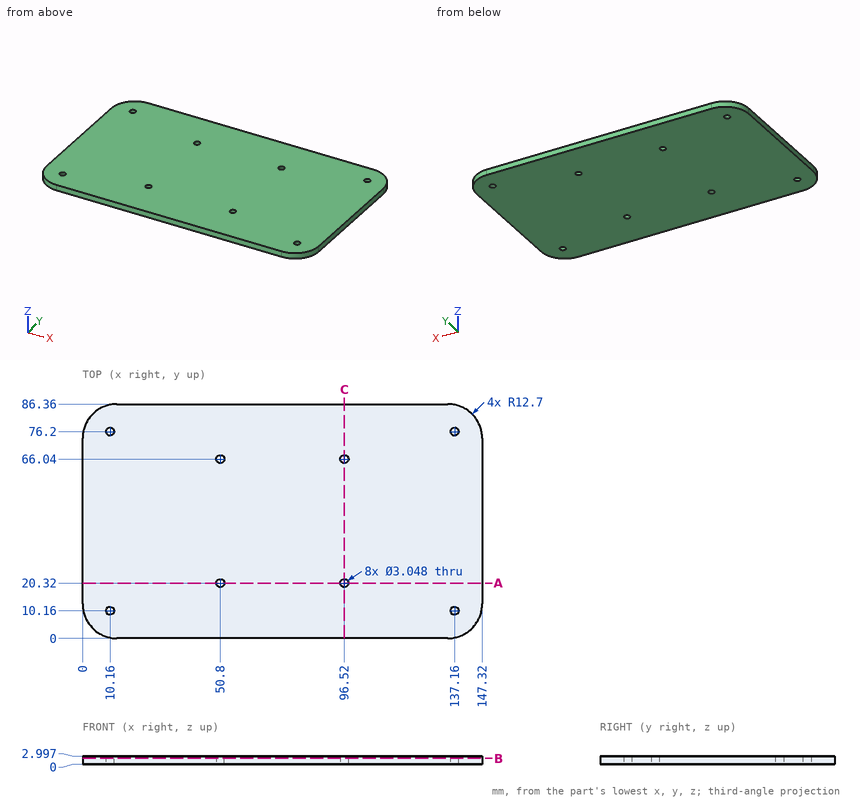
Answer from the drawing. Dimensions are ordinates in mm from the lowest x, y and z of the part. Round coordinates to 2 decimals unless told otherwise and drop trailing zeros. Loops run counter-clockwise (first coordinate to the right, second up) from the corner with the lowest first, then second, coordinate; pieces in that order, holes last.
1) A cutting plane is placed at B-B on z = 2.2. Give the number of separate pieces and of enclosed holes in the cut face, plus the area to 3 significant figures.
Outcome:
separate pieces: 1
enclosed holes: 8
area: 12,500 mm2
2) Given P1, Ø2.5, axis at x = 10.16, y = 76.2, coming from the +Z side; P2, Ø4, axis at x = 50.8, y = 66.04, coming from the -Z side, each flat-ended and moving along its own axis, determine where each tip first touches the part or whether it passes through.
Outcome:
P1: passes through
P2: stops at z = 0
3) Consider line 1 (Y direction, x = 50.8, z = 0.8); line 2 (X direction, y = 66.04, z = 1.5); line 3 (Y direction, x = 137, z = 1.85) (1 decimal). Determine where each line is inside the solid, lowest interval first.
Outcome:
line 1: y = 0 to 18.8, 21.84 to 64.52, 67.56 to 86.36
line 2: x = 0 to 49.28, 52.32 to 95, 98.04 to 147.32
line 3: y = 0.2 to 8.6, 11.7 to 74.7, 77.7 to 86.1
4) A cutting plane is placed at A-A on y = 20.32. Determine the outline of the cut face in (x, z), plus the area to 3 significant figures.
Outcome:
outline: (0, 0) - (49.28, 0) - (49.28, 3) - (0, 3) - close; (52.32, 0) - (95, 0) - (95, 3) - (52.32, 3) - close; (98.04, 0) - (147.32, 0) - (147.32, 3) - (98.04, 3) - close
area: 423 mm2
5) A cutting plane is placed at C-C on x = 96.52. Determine the outline of the cut face in (y, z).
Outcome:
outline: (0, 0) - (18.8, 0) - (18.8, 3) - (0, 3) - close; (21.84, 0) - (64.52, 0) - (64.52, 3) - (21.84, 3) - close; (67.56, 0) - (86.36, 0) - (86.36, 3) - (67.56, 3) - close
